Geometry check sheet. Reference: the model listing, model coordinates, mm. A direction names the side the tool comes from. Round coordinates to 2 decimals unless told otherwise and drop trailing zeros. Loops run counter-clockwise (first coordinate to the right, second up) from the corner with the lowest first, then second, coordinate; pieces in that order, holes last. Notation, with made-up numbers: M -7.5,-39.75 L 31.5,-39.75 A5 cw 31.5,-35.75 Z; hole C -24.5,33 d11. An arc over 180 degrees is marked long. Use one line per item in the form item = value. Start each with the question number.
1. Cross-section at A-A (x = 288). Record the boundary of the cut face in (y, z).
2. Go/stop test with flat-tipped pins: pin 1 (14.5 mm diameter, centred on x = 86.5, z = 10, fed in from -Y); pin 2 (24 mm diameter, centred on y = -1, z = 40.5, fed in from -X). Record where each tip stops, or that it passes through.
3. Set-up check for faces 4 (the flat face through (387.261, 27.003, -46.753)), 5 (the flat face through (381, 0, 0)), 6 (the flat face through (4, 25.4, 0)): record each of +Z, -Z, +X, -X, +Y, -Y from which the full face is reachable in a straight line by a thin tool's end or side.
4. Material ranges on line 1 (Y direction, x = 340.5, z = -9); line 2 (X direction, y = 39, z = 14), recorded low to high.
5. Cross-section at B-B (y = 75.5). Record the boundary of the cut face in (x, z).
6. Draft check along Y on faces 1 (the cylindrical face through (287.845, 108.482, -2.432)), 2 (the flat face through (387.26, -27.05, -47.36)), 3 (the flat face through (-19.05, 3.5, 45.1)). Enter one of: pulls with the +Y half, pulls with the -Y half, needs draft (parallel to the pull), parting line crosses it, or undercut.
7. Cross-section at C-C (z = -46.5). Record the boundary of the cut face in (x, y), then the cut area to 3 significant figures.
8. Cross-section at D-D (x = -139). Record the boundary of the cut face in (y, z).
```python
from build123d import *

# Parameters (mm, degrees)
SKETCH1_W           = 50.8
SKETCH1_H           = 50.8
SKETCH1_W_2         = 47.625
SKETCH1_H_2         = 47.625
BOSS_EXTRUDE1_DEPTH = 381
SKETCH2_R           = 11.598122223
SKETCH2_R_2         = 10.010622223
BOSS_EXTRUDE2_DEPTH = 19.05
SKETCH3_W           = 6.35
SKETCH3_H           = 50.8
BOSS_EXTRUDE3_DEPTH = 101.092
SKETCH7_R           = 12.7
BOSS_EXTRUDE4_DEPTH = 12.7


with BuildPart() as part:
    # Sketch1 → Boss-Extrude1 (new body, symmetric)
    with BuildSketch(Plane(origin=(0, 0, 0), x_dir=(0, 0, -1), z_dir=(1, 0, 0))):
        Rectangle(SKETCH1_W, SKETCH1_H)
        Rectangle(SKETCH1_W_2, SKETCH1_H_2, mode=Mode.SUBTRACT)
    extrude(amount=BOSS_EXTRUDE1_DEPTH, both=True)

    # Sketch2 → Boss-Extrude2 (add, symmetric)
    with BuildSketch(Plane(origin=(0, 0, 0), x_dir=(0, 0, -1), z_dir=(1, 0, 0))):
        with Locations((-35.410622223, 0)):
            Circle(SKETCH2_R)
        with Locations((-35.410622223, 0)):
            Circle(SKETCH2_R_2, mode=Mode.SUBTRACT)
    extrude(amount=BOSS_EXTRUDE2_DEPTH, both=True)

    # Sketch3 → Boss-Extrude3 (add)
    with BuildSketch(Plane(origin=(0, 25.4, 0), x_dir=(1, 0, 0), z_dir=(0, 1, 0))):
        with Locations((-277.368, 0)):
            Rectangle(SKETCH3_W, SKETCH3_H)
        with Locations((277.368, 0)):
            Rectangle(SKETCH3_W, SKETCH3_H)
    extrude(amount=BOSS_EXTRUDE3_DEPTH)

    # Sketch5 → Revolve1 (revolve)
    with BuildSketch(Plane.XY):
        with BuildLine():
            Line((280.543, 108.966), (294.944477372, 108.966))
            ThreePointArc((294.944477372, 108.966), (309.230001873, 114.883257994), (318.643, 102.616))
            Line((318.643, 102.616), (280.543, 102.616))
            Line((280.543, 102.616), (280.543, 108.966))
        make_face()
    revolve1 = revolve(axis=Axis((280.543, 102.616, 0), (1, 0, 0)))

    # Mirror1: Revolve1 across plane
    add(revolve1.mirror(Plane(origin=(0, 0, 0), x_dir=(0, 0, 1), z_dir=(1, 0, 0))))

    # Sketch6 → Revolve2 (revolve)
    with BuildSketch(Plane(origin=(0, 0, 0), x_dir=(0, 0, -1), z_dir=(1, 0, 0))):
        with BuildLine():
            Line((-6.35, -25.4), (0, -25.4))
            Line((0, -25.4), (0, -63.5))
            ThreePointArc((0, -63.5), (-12.267257994, -54.087001873), (-6.35, -39.801477372))
            Line((-6.35, -39.801477372), (-6.35, -25.4))
        make_face()
    revolve(axis=Axis((0, -25.4, 0), (0, -1, 0)))

    # Sketch7 → Boss-Extrude4 (add)
    with BuildSketch(Plane(origin=(381, 0, 0), x_dir=(0, 0, -1), z_dir=(1, 0, 0))):
        with BuildLine():
            Line((68.713128758, -28.652376301), (25.4, -25.4))
            Line((25.4, -25.4), (-25.4, -25.4))
            Line((-25.4, -25.4), (-25.4, 25.4))
            Line((-25.4, 25.4), (25.4, 25.4))
            Line((25.4, 25.4), (68.713128758, 28.6523763))
            ThreePointArc((68.713128758, 28.6523763), (99.597672127, 0), (68.713128758, -28.652376301))
        make_face()
        with Locations((70.86463137, 0)):
            Circle(SKETCH7_R, mode=Mode.SUBTRACT)
    boss_extrude4 = extrude(amount=BOSS_EXTRUDE4_DEPTH)

    # Mirror2: Boss-Extrude4 across plane
    add(boss_extrude4.mirror(Plane(origin=(0, 0, 0), x_dir=(0, 0, 1), z_dir=(1, 0, 0))))


solid = part.part
```
Reported:
q1.outline = M -25.4,-25.4 L 25.4,-25.4 L 25.4,25.4 L -25.4,25.4 Z; C 102.62,0 d12.7; hole M -23.81,-23.81 L 23.81,-23.81 L 23.81,23.81 L -23.81,23.81 Z
q2.pin_1 = -25.4
q2.pin_2 = -19.05
q3.face_4 = +Z, +X, -X, +Y
q3.face_5 = none
q3.face_6 = +Z, -Z, +Y
q4.line_1 = -25.4 to -23.81, 23.81 to 25.4
q4.line_2 = -280.54 to -274.19, 274.19 to 280.54
q5.outline = M -280.54,-25.4 L -274.19,-25.4 L -274.19,25.4 L -280.54,25.4 Z; M 274.19,-25.4 L 280.54,-25.4 L 280.54,25.4 L 274.19,25.4 Z
q6.face_1 = undercut
q6.face_2 = pulls with the -Y half
q6.face_3 = needs draft
q7.outline = M -393.7,-26.98 L -381,-26.98 L -381,26.98 L -393.7,26.98 Z; M 381,-26.98 L 393.7,-26.98 L 393.7,26.98 L 381,26.98 Z
q7.area = 1,370 mm²
q8.outline = M -25.4,-25.4 L 25.4,-25.4 L 25.4,25.4 L -25.4,25.4 Z; hole M -23.81,-23.81 L 23.81,-23.81 L 23.81,23.81 L -23.81,23.81 Z
